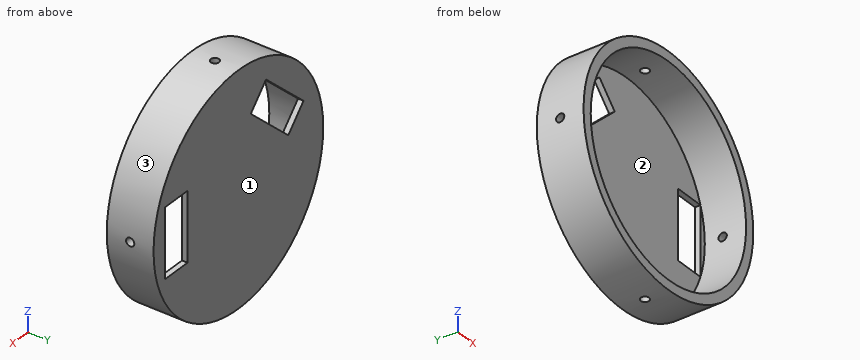
```python
from build123d import *

# Parameters (mm, degrees)
SKETCH1_R               = 41.5
SKETCH1_R_2             = 38
BOSS_EXTRUDE1_DEPTH     = 15
SKETCH2_R               = 41.5
BOSS_EXTRUDE2_DEPTH     = 2
SKETCH3_W               = 11
SKETCH3_H               = 25
CUT_EXTRUDE1_DEPTH      = 3
SKETCH4_R               = 1.5
CUT_EXTRUDE2_DEPTH      = 80
CUT_EXTRUDE2_DEPTH_BACK = 80
SKETCH5_R               = 1.5
CUT_EXTRUDE4_DEPTH      = 80
CUT_EXTRUDE4_DEPTH_BACK = 80


with BuildPart() as part:
    # Sketch1 → Boss-Extrude1 (new body)
    with BuildSketch(Plane(origin=(0, 0, 0), x_dir=(1, 0, 0), z_dir=(0, 1, 0))):
        Circle(SKETCH1_R)
        Circle(SKETCH1_R_2, mode=Mode.SUBTRACT)
    extrude(amount=BOSS_EXTRUDE1_DEPTH)

    # Sketch2 → Boss-Extrude2 (add)
    with BuildSketch(Plane(origin=(0, 15, 0), x_dir=(1, 0, 0), z_dir=(0, 1, 0))):
        Circle(SKETCH2_R)
    extrude(amount=BOSS_EXTRUDE2_DEPTH)

    # Sketch3 → Cut-Extrude1 (cut)
    with BuildSketch(Plane(origin=(0, 17, 0), x_dir=(1, 0, 0), z_dir=(0, 1, 0))):
        Polygon((-6.046682172, -23.124314263), (-13.51904975, -31.19671928), (-31.86542479, -14.214065692), (-24.393057211, -6.141660674), align=None)
        with Locations((30.385233732, 0)):
            Rectangle(SKETCH3_W, SKETCH3_H)
    extrude(amount=-CUT_EXTRUDE1_DEPTH, mode=Mode.SUBTRACT)

    # Sketch4 → Cut-Extrude2 (cut, two sides)
    with BuildSketch(Plane.XY) as cut_extrude2_sk:
        with Locations((0, 8.5)):
            Circle(SKETCH4_R)
    extrude(amount=CUT_EXTRUDE2_DEPTH, mode=Mode.SUBTRACT)
    extrude(cut_extrude2_sk.sketch, amount=-CUT_EXTRUDE2_DEPTH_BACK, mode=Mode.SUBTRACT)

    # Sketch5 → Cut-Extrude4 (cut, two sides)
    with BuildSketch(Plane(origin=(0, 0, 0), x_dir=(0, 0, -1), z_dir=(1, 0, 0))) as cut_extrude4_sk:
        with Locations((0, 8.5)):
            Circle(SKETCH5_R)
    extrude(amount=CUT_EXTRUDE4_DEPTH, mode=Mode.SUBTRACT)
    extrude(cut_extrude4_sk.sketch, amount=-CUT_EXTRUDE4_DEPTH_BACK, mode=Mode.SUBTRACT)


solid = part.part
```
Can you work these out from the model? Positions are in its coordinate system, mm. Face numbers are marked on the shaded views. Coordinates: 2 decimals unless noted, no trailing zeros. Loops run counter-clockwise (first coordinate to the right, second up) from the corner with the lowest first, then second, coordinate; pieces in that order, holes last. Notation, with made-up numbers: M 20.5,65 L 64.5,65 A19 ccw 64.5,87 Z; hole C -27.5,73 d7. An arc over 180 degrees is marked long. Put each result on its own line as item: value. Start each with the question number.
(1) I need wall thicknesses on probe 1 along Y at (x, z) = (-39.75, 0); probe 2 along X at (y, z) = (5, 0). Which ranges of each line are inside material? Lowest first, please.
(2) Will these pins go through, and if not, where does the flat tip stop? pin 1 Ø10 at (y, z) = (3.5, -13.5) entering from +X; pin 2 Ø4 at (y, z) = (2, -25) entering from +X; pin 3 Ø6 at (y, z) = (9, -11) entering from -X; pin 4 Ø1.8 at (x, y) = (0, 8.5) entering from +Z.
(3) Imagine slicing it at D-D on y = 8.5. List the corners of the cut face in (x, z) for me, and give its area (3 significant figures).
(4) Imagine slicing it at C-C on x = -23. List the corners of the cut face in (y, z) for me.
(5) Imagine slicing it at A-A on x = 0. List the corners of the cut face in (y, z) for me, and give its area (3 significant figures).
(6) We'd pull the mould along X, two halves only. Please class the marked faces 1, 2 and 3: +X half, -X half, draft (parallel to the pull), parting line (faces both ways), or undercut.
(7) Imagine slicing it at B-B on z = 0. List the corners of the cut face in (x, y) for me.
Worked answers:
1. probe 1: y = 0 to 7, 10 to 17
1. probe 2: x = -41.5 to -38, 38 to 41.5
2. pin 1: stops at x = 40.62
2. pin 2: stops at x = 34.54
2. pin 3: stops at x = -40.72
2. pin 4: passes through
3. outline: M -41.47,-1.5 A41.5 ccw -1.5,-41.47 L -1.5,-37.97 A38 cw -37.97,-1.5 Z; M -41.47,1.5 L -37.97,1.5 A38 cw -1.5,37.97 L -1.5,41.47 A41.5 ccw Z; M 1.5,-41.47 A41.5 ccw 41.47,-1.5 L 37.97,-1.5 A38 cw 1.5,-37.97 Z; M 1.5,37.97 A38 cw 37.97,1.5 L 41.47,1.5 A41.5 ccw 1.5,41.47 Z
3. area: 832 mm2
4. outline: M 0,-34.54 L 17,-34.54 L 17,7.43 L 15,7.43 L 15,-30.25 L 0,-30.25 Z; M 0,30.25 L 15,30.25 L 15,22.42 L 17,22.42 L 17,34.54 L 0,34.54 Z
5. outline: M 0,-41.5 L 7,-41.5 L 7,-38 L 0,-38 Z; M 0,38 L 7,38 L 7,41.5 L 0,41.5 Z; M 10,-41.5 L 17,-41.5 L 17,41.5 L 10,41.5 L 10,38 L 15,38 L 15,-38 L 10,-38 Z
5. area: 250 mm2
6. face 1: draft
6. face 2: undercut
6. face 3: parting line
7. outline: M -41.5,0 L -38,0 L -38,7 L -41.5,7 Z; M -41.5,10 L -38,10 L -38,15 L 24.89,15 L 24.89,17 L -41.5,17 Z; M 35.89,15 L 38,15 L 38,10 L 41.5,10 L 41.5,17 L 35.89,17 Z; M 38,0 L 41.5,0 L 41.5,7 L 38,7 Z
